from build123d import *

# Parameters (mm, degrees)
SKETCH_1_W              = 200
SKETCH_1_H              = 200
EXTRUDE_1_DEPTH         = 3
SKETCH_2_R              = 1.5
CUT_EXTRUDE_2_DEPTH     = 10
CUT_EXTRUDE_3_DEPTH     = 10
SKETCH_6_R              = 1.55
CUT_EXTRUDE_3_1_1_DEPTH = 10
CUT_EXTRUDE_6_REACH     = 111.495
SKETCH_11_R             = 1.5
CUT_EXTRUDE_22_5_REACH  = 111.495
SKETCH_4_R              = 11.25
FILLET_1_R              = 1
SKETCH_12_W             = 40
SKETCH_12_H             = 3
EXTRUDE_2_DEPTH         = 75
FILLET_2_R              = 7
SKETCH_13_R             = 1.55
CUT_EXTRUDE_3_1_DEPTH   = 10
SKETCH_16_R             = 1.55
SKETCH_16_R_2           = 6.5
CUT_EXTRUDE_6242_DEPTH  = 10
SKETCH_18_W             = 87.5
SKETCH_18_H             = 3
EXTRUDE_3_DEPTH         = 20.5
SKETCH_19_W             = 87.5
SKETCH_19_H             = 3
EXTRUDE_4_DEPTH         = 20.5
SKETCH_7_R              = 1.55
CUT_EXTRUDE_7_DEPTH     = 20.5
FILLET_3_R              = 8


with BuildPart() as part:
    # 草图1 → 凸台-拉伸1 (new body)
    with BuildSketch(Plane(origin=(0, 0, 0), x_dir=(1, 0, 0), z_dir=(0, 1, 0))):
        Rectangle(SKETCH_1_W, SKETCH_1_H)
    extrude(amount=EXTRUDE_1_DEPTH)

    # 草图2 → 切除-拉伸2 (cut)
    with BuildSketch(Plane(origin=(0, 3, 0), x_dir=(1, 0, 0), z_dir=(0, 1, 0))):
        with Locations(Location((29.5, 9.5, 0), (0, 0, 270))):
            Circle(SKETCH_2_R)
        with Locations(Location((21.5, 0, 0), (0, 0, 270))):
            Circle(SKETCH_2_R)
        with Locations(Location((29.5, -9.5, 0), (0, 0, 270))):
            Circle(SKETCH_2_R)
        with Locations(Location((37.5, 0, 0), (0, 0, 270))):
            Circle(SKETCH_2_R)
        with Locations(Location((-29.5, -9.5, 0), (0, 0, 270))):
            Circle(SKETCH_2_R)
        with Locations(Location((-37.5, 0, 0), (0, 0, 270))):
            Circle(SKETCH_2_R)
        with Locations(Location((-21.5, 0, 0), (0, 0, 270))):
            Circle(SKETCH_2_R)
        with Locations(Location((-29.5, 9.5, 0), (0, 0, 270))):
            Circle(SKETCH_2_R)
    extrude(amount=-CUT_EXTRUDE_2_DEPTH, mode=Mode.SUBTRACT)

    # 草图5 → 切除-拉伸3 (cut)
    with BuildSketch(Plane(origin=(0, 3, 0), x_dir=(1, 0, 0), z_dir=(0, 1, 0))):
        with BuildLine():
            Line((-100, -100), (-44.5, -100))
            Line((-44.5, -100), (-44.5, 0))
            ThreePointArc((-44.5, 0), (-40.212142643, 10.5), (-29.8, 14.9969997))
            ThreePointArc((-29.8, 14.9969997), (-22.858571571, 17.9949995), (-20, 24.9949995))
            Line((-20, 24.9949995), (-20, 47.5))
            Line((-20, 47.5), (0, 47.5))
            Line((0, 47.5), (20, 47.5))
            Line((20, 47.5), (20, 24.9949995))
            ThreePointArc((20, 24.9949995), (22.858571571, 17.9949995), (29.8, 14.9969997))
            ThreePointArc((29.8, 14.9969997), (40.212142643, 10.5), (44.5, 0))
            Line((44.5, 0), (44.5, -100))
            Line((44.5, -100), (100, -100))
            Line((100, -100), (100, 100))
            Line((100, 100), (-100, 100))
            Line((-100, 100), (-100, -100))
        make_face()
    extrude(amount=-CUT_EXTRUDE_3_DEPTH, mode=Mode.SUBTRACT)

    # 草图6 → φ3.1通孔1 (cut)
    with BuildSketch(Plane.XZ):
        with Locations(Location((-15, -42.5, 0), (0, 0, 270))):
            Circle(SKETCH_6_R)
        with Locations(Location((-15, -27.5, 0), (0, 0, 270))):
            Circle(SKETCH_6_R)
        with Locations(Location((15, -27.5, 0), (0, 0, 90))):
            Circle(SKETCH_6_R)
        with Locations(Location((15, -42.5, 0), (0, 0, 90))):
            Circle(SKETCH_6_R)
    extrude(amount=-CUT_EXTRUDE_3_1_1_DEPTH, mode=Mode.SUBTRACT)

    # 草图11 → 切除-拉伸6 (cut, up to next)
    with BuildSketch(Plane(origin=(0, 3, 0), x_dir=(1, 0, 0), z_dir=(0, 1, 0)), mode=Mode.PRIVATE) as cut_extrude_6_sk1:
        with BuildLine():
            Line((44.5, -17.5), (44.5, -100))
            Line((44.5, -100), (101.133062566, -100))
            Line((101.133062566, -100), (101.133062566, 47.5))
            Line((101.133062566, 47.5), (20, 47.5))
            Line((20, 47.5), (20, 7.5))
            Line((20, 7.5), (19, 7.5))
            ThreePointArc((19, 7.5), (18.292893219, 7.207106781), (18, 6.5))
            Line((18, 6.5), (18, -4))
            ThreePointArc((18, -4), (20.48959236, -10.01040764), (26.5, -12.5))
            Line((26.5, -12.5), (39.5, -12.5))
            Line((39.5, -12.5), (44.5, -12.5))
            Line((44.5, -12.5), (44.5, -17.5))
        make_face()
        with Locations((29.5, -9.5)):
            Circle(SKETCH_11_R, mode=Mode.SUBTRACT)
        with Locations((21.5, 0)):
            Circle(SKETCH_11_R, mode=Mode.SUBTRACT)
    cut_extrude_6_tool1 = extrude(cut_extrude_6_sk1.sketch, amount=-CUT_EXTRUDE_6_REACH, mode=Mode.PRIVATE) & part.part
    # 草图11 → 切除-拉伸6 (cut, up to next)
    with BuildSketch(Plane(origin=(0, 3, 0), x_dir=(1, 0, 0), z_dir=(0, 1, 0)), mode=Mode.PRIVATE) as cut_extrude_6_sk2:
        with BuildLine():
            Line((-44.5, -17.5), (-44.5, -100))
            Line((-44.5, -100), (-101.133062566, -100))
            Line((-101.133062566, -100), (-101.133062566, 47.5))
            Line((-101.133062566, 47.5), (-20, 47.5))
            Line((-20, 47.5), (-20, 7.5))
            Line((-20, 7.5), (-19, 7.5))
            ThreePointArc((-19, 7.5), (-18.292893219, 7.207106781), (-18, 6.5))
            Line((-18, 6.5), (-18, -4))
            ThreePointArc((-18, -4), (-20.48959236, -10.01040764), (-26.5, -12.5))
            Line((-26.5, -12.5), (-39.5, -12.5))
            Line((-39.5, -12.5), (-44.5, -12.5))
            Line((-44.5, -12.5), (-44.5, -17.5))
        make_face()
    cut_extrude_6_tool2 = extrude(cut_extrude_6_sk2.sketch, amount=-CUT_EXTRUDE_6_REACH, mode=Mode.PRIVATE) & part.part
    add(cut_extrude_6_tool1.solids().sort_by_distance((66.686037, 3, 19.669577))[0], mode=Mode.SUBTRACT)
    add(cut_extrude_6_tool2.solids().sort_by_distance((-66.626911, 3, 19.648158))[0], mode=Mode.SUBTRACT)

    # 草图4 → φ22.5落弹孔 (cut, up to next)
    with BuildSketch(Plane(origin=(0, 3, 0), x_dir=(1, 0, 0), z_dir=(0, 1, 0)), mode=Mode.PRIVATE) as cut_extrude_22_5_sk1:
        with Locations(Location((0, -29, 0), (0, 0, 270))):
            Circle(SKETCH_4_R)
    cut_extrude_22_5_tool1 = extrude(cut_extrude_22_5_sk1.sketch, amount=-CUT_EXTRUDE_22_5_REACH, mode=Mode.PRIVATE) & part.part
    add(cut_extrude_22_5_tool1.solids().sort_by_distance((0, 3, 29))[0], mode=Mode.SUBTRACT)

    # 圆角1
    fillet_1_edges = [part.edges().sort_by_distance(p)[0] for p in [
        (-20, 1.5, -7.5),
        (20, 1.5, -7.5),
    ]]
    fillet(fillet_1_edges, radius=FILLET_1_R - 0.0001)  # a hair under: the kernel refuses the full size

    # 草图12 → 凸台-拉伸2 (add)
    with BuildSketch(Plane(origin=(0, 0, -47.5), x_dir=(-1, 0, 0), z_dir=(0, 0, -1))):
        with Locations((0, 1.5)):
            Rectangle(SKETCH_12_W, SKETCH_12_H)
    extrude(amount=EXTRUDE_2_DEPTH)

    # 圆角2
    fillet_2_edges = [part.edges().sort_by_distance(p)[0] for p in [
        (20, 1.5, -122.5),
        (-20, 1.5, -122.5),
    ]]
    fillet(fillet_2_edges, radius=FILLET_2_R)

    # 草图13 → φ3.1通孔 (cut)
    with BuildSketch(Plane(origin=(0, 3, 0), x_dir=(1, 0, 0), z_dir=(0, 1, 0))):
        with Locations(Location((-8.625, 113.5, 0), (0, 0, 270))):
            Circle(SKETCH_13_R)
        with Locations(Location((8.625, 113.5, 0), (0, 0, 270))):
            Circle(SKETCH_13_R)
        with Locations(Location((8.625, 73.5, 0), (0, 0, 270))):
            Circle(SKETCH_13_R)
        with Locations(Location((-8.625, 73.5, 0), (0, 0, 270))):
            Circle(SKETCH_13_R)
    extrude(amount=-CUT_EXTRUDE_3_1_DEPTH, mode=Mode.SUBTRACT)

    # 草图16 → Cut-Extrude 6242 (cut)
    with BuildSketch(Plane(origin=(0, 3, 0), x_dir=(1, 0, 0), z_dir=(0, 1, 0))):
        with Locations(Location((0, -62.75, 0), (0, 0, 270))):
            Circle(SKETCH_16_R)
        with Locations(Location((-8.227241336, -48.5, 0), (0, 0, 270))):
            Circle(SKETCH_16_R)
        with Locations(Location((8.227241336, -48.5, 0), (0, 0, 270))):
            Circle(SKETCH_16_R)
        with Locations(Location((0, -53.25, 0), (0, 0, 270))):
            Circle(SKETCH_16_R_2)
    extrude(amount=-CUT_EXTRUDE_6242_DEPTH, mode=Mode.SUBTRACT)

    # 草图18 → 凸台-拉伸3 (add)
    with BuildSketch(Plane.ZY.offset(44.5)):
        with Locations((56.25, 1.5)):
            Rectangle(SKETCH_18_W, SKETCH_18_H)
    extrude(amount=EXTRUDE_3_DEPTH)

    # 草图19 → 凸台-拉伸4 (add)
    with BuildSketch(Plane(origin=(44.5, 0, 0), x_dir=(0, 0, -1), z_dir=(1, 0, 0))):
        with Locations((-56.25, 1.5)):
            Rectangle(SKETCH_19_W, SKETCH_19_H)
    extrude(amount=EXTRUDE_4_DEPTH)

    # 草图7 → 切除-拉伸7 (cut)
    with BuildSketch(Plane(origin=(0, 3, 0), x_dir=(1, 0, 0), z_dir=(0, 1, 0))):
        with Locations(Location((-61, -28.5, 0), (0, 0, 270))):
            Circle(SKETCH_7_R)
        with Locations(Location((-61, -50.5, 0), (0, 0, 270))):
            Circle(SKETCH_7_R)
        with Locations(Location((61, -28.5, 0), (0, 0, 270))):
            Circle(SKETCH_7_R)
        with Locations(Location((61, -50.5, 0), (0, 0, 270))):
            Circle(SKETCH_7_R)
    extrude(amount=-CUT_EXTRUDE_7_DEPTH, mode=Mode.SUBTRACT)

    # 圆角3
    fillet_3_edges = [part.edges().sort_by_distance(p)[0] for p in [
        (-65, 1.5, 12.5),
        (65, 1.5, 12.5),
    ]]
    fillet(fillet_3_edges, radius=FILLET_3_R)


solid = part.part
Build history of the part. All positions in model axes, mm. A direction names the side the tool comes from. Round coordinates to 2 decimals unless told otherwise and drop trailing zeros. Write each loop counter-clockwise with the first axis right and the second up, starting at its lowest first coordinate (ties: lowest second). Pieces come first, ordered by that corner, then holes. Notation, with made-up numbers: M 84.5,61 L 89.5,61 A15 ccw 89.5,77 Z; hole C -18,-10 d10. An arc over 180 degrees is marked long. Answer as a JSON object with one key per item and string values. Group by question number.
(1) Flat gauge pins, fed straight in: pin 1 (1 mm diameter, centred on x = -23.5, y = 2, fed in from -Z); pin 2 (0.9 mm diameter, centred on x = 35.5, y = 2, fed in from -Z); pin 3 (0.9 mm diameter, centred on y = 2, z = 0.5, fed in from -X). Where does each tip first touch, or does it go through?
(2) Cut at C-C (y = 2.55). Give the number of separate pieces and of enclosed holes in the cut face, and give its area (3 significant figures).
(3) Drill centre lines: L1, parallel to X at y = 1.55, z = -73.5 (3 decimals); L2, parallel to X at y = 1.35, z = 28.5; L3, parallel to X at y = 0.8, z = 48.5. Where is each one in solid material? Low to high.
(4) Cut at B-B (z = -56). Give the cut face in (x, y), and give its area (3 significant figures).
(5) Which spindle directions (+Z, -Z, +X, -X, +Y, -Y) get a long thin tool onto all of the face, cutting with end or side? Do faces 4 (the cylindrical face through (-20.42, 1.52, 9.94)), 5 (the cylindrical face through (-62.719, 1.521, 14.906)). Say none if no direction does.
(6) Mould opens along X. For faces 1 (the cylindrical face through (-18, 1.5, -120.4)), 2 (the cylindrical face through (20.42, 1.52, 9.94)), 3 (the cylindrical face through (9.486, 1.521, 35.048)) say: pulls with the +X half, pulls with the -X half, needs draft (parallel to the pull), parting line crosses it, or undercut.
(7) Cut at A-A (x = -35.5). Give the cut face in (y, z), and give its area (4 significant figures).
Responses:
{
 "1": {"pin 1": "stops at z = 11.75", "pin 2": "stops at z = 12.5", "pin 3": "stops at x = -18"},
 "2": {"separate pieces": "1", "enclosed holes": "17", "area": "16,000 mm2"},
 "3": {"L1": "x = -20 to -10.175, -7.075 to 7.075, 10.175 to 20", "L2": "x = -65 to -62.55, -59.45 to -11.24, 11.24 to 59.45, 62.55 to 65", "L3": "x = -65 to -9.78, -6.68 to -4.44, 4.44 to 6.68, 9.78 to 65"},
 "4": {"outline": "M -20,0 L 20,0 L 20,3 L -20,3 Z", "area": "120 mm2"},
 "5": {"face 4": "-X, +Y, -Y", "face 5": "-Z, -X, +Y, -Y"},
 "6": {"face 1": "pulls with the -X half", "face 2": "pulls with the +X half", "face 3": "undercut"},
 "7": {"outline": "M 0,12.5 L 3,12.5 L 3,100 L 0,100 Z", "area": "262.5 mm2"}
}
